Design review of the part shown in the three views and the two pictorial views. Dimensions are in mm from the part's minimum x, y and z. A direction names the side the tool comes from. Give positions to 0.01 mm unless a question says otherwise; leave off trailing zeros. Order: outer loops, then holes, each group sorted by start corner. A loop starts at its lowest first (then second) coordinate and runs counter-clockwise, first axis right, second up.
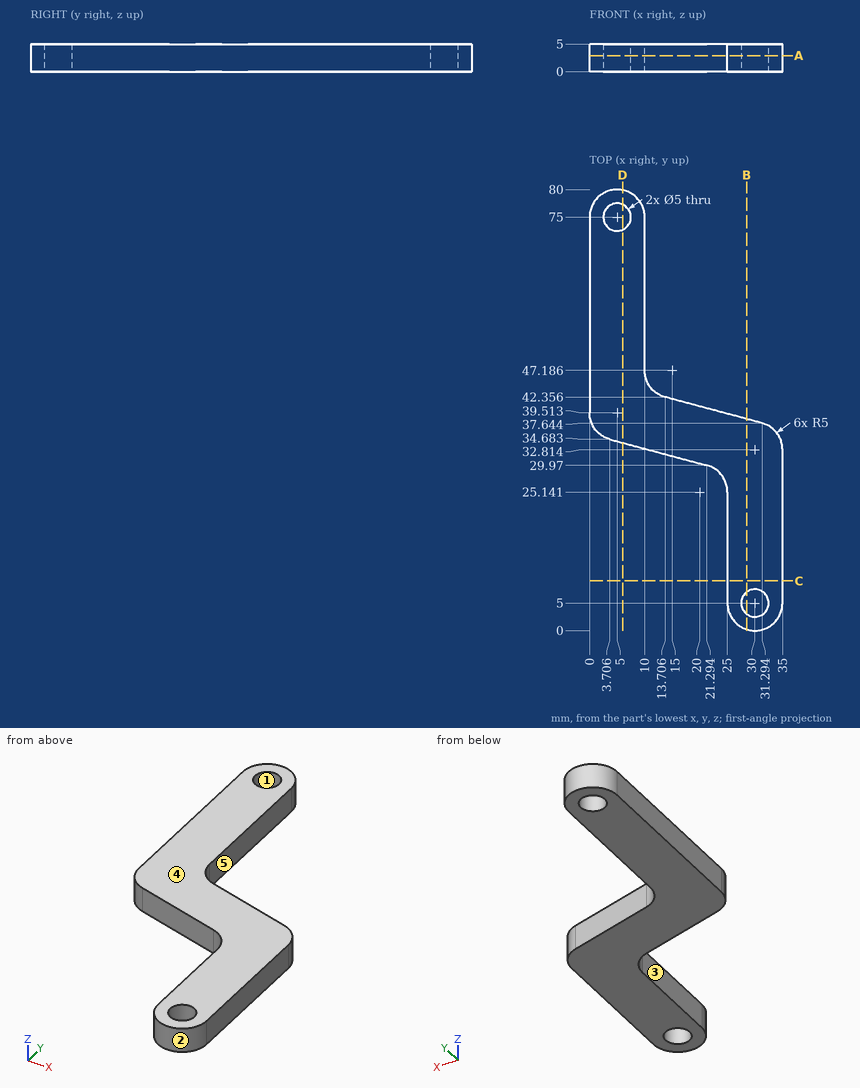
1) Draft analysis for pull direction X (two halves, no side actions). For the marked faces 1, 2 and 3, state which applies: +X half, -X half, draft (parallel to the pull), parting line (faces both ways), or undercut.
Answer sheet:
face 1: undercut
face 2: parting line
face 3: -X half
2) We need section C-C on y = 9. Give the boundary of the cut face in (x, z), then the cut area to 3 significant figures.
Answer sheet:
outline: (25, 0) - (35, 0) - (35, 5) - (25, 5) - close
area: 50.0 mm2
3) Tool access review of the marked faces 4 and 5: name each direction out of +Z, -Z, +X, -X, +Y, -Y from which nothing blocks a thin tool from reaching the whole face with its end or side.
Answer sheet:
face 4: +Z, +X, -X, +Y, -Y
face 5: +Z, -Z, +X, +Y
4) We need section B-B on x = 28.5. Give the boundary of the cut face in (y, z), then the cut area to 3 significant figures.
Answer sheet:
outline: (0.23, 0) - (3, 0) - (3, 5) - (0.23, 5) - close; (7, 0) - (38.39, 0) - (38.39, 5) - (7, 5) - close
area: 171 mm2
5) Clearance check with flat-ended pins moving along their axes: pin 1 (1 mm diameter, centred on x = 14, z = 2.5, fed in from -Y); pin 2 (1.5 mm diameter, centred on y = 57.5, z = 3, fed in from +X); pin 3 (1 mm diameter, centred on y = 36.5, z = 2.5, fed in from -X). State where each tip first meets the part, or that it passes through.
Answer sheet:
pin 1: stops at y = 31.79
pin 2: stops at x = 10
pin 3: stops at x = 0.68
6) We need section D-D on x = 6. Give the boundary of the cut face in (y, z).
Answer sheet:
outline: (34.07, 0) - (72.71, 0) - (72.71, 5) - (34.07, 5) - close; (77.29, 0) - (79.9, 0) - (79.9, 5) - (77.29, 5) - close
7) We need section A-A on z = 2.9. Give the boundary of the cut face in (x, y), then the cut area to 3 significant figures.
Answer sheet:
outline: (0, 39.51) arc R5 ccw to (3.71, 34.68) - (21.29, 29.97) arc R5 cw to (25, 25.14) - (25, 5) arc R5 ccw to (35, 5) - (35, 32.81) arc R5 ccw to (31.29, 37.64) - (13.71, 42.36) arc R5 cw to (10, 47.19) - (10, 75) arc R5 ccw to (0, 75) - close; hole circle Ø5 at (5, 75); hole circle Ø5 at (30, 5)
area: 931 mm2
8) To check wall thickness, follow line 1 (X direction, y = 75, z = 2.3); line 2 (Y direction, x = 5, z = 2.1); line 3 (Y direction, x = 4, z = 1.75) (1 decimal). State the ranges of each line that lie inside material, in increasing order.
Answer sheet:
line 1: x = 0 to 2.5, 7.5 to 10
line 2: y = 34.34 to 72.5, 77.5 to 80
line 3: y = 34.6 to 72.7, 77.3 to 79.9
